```python
from build123d import *

# Parameters (mm, degrees)
BOSS_EXTRUDE1_DEPTH      = 5
BOSS_EXTRUDE1_DEPTH_BACK = 52.601
BOSS_EXTRUDE2_DEPTH      = 5
SKETCH3_W                = 4
SKETCH3_H                = 6
F_8_CLEARANCE_HOLE1_D    = 4.4958
CHAMFER1_SIZE            = 4
CUT_EXTRUDE7_DEPTH       = 189.558951211
BOSS_EXTRUDE10_START     = -5
BOSS_EXTRUDE10_DEPTH     = 5
CHAMFER4_SIZE            = 1


with BuildPart() as part:
    # Sketch1 → Boss-Extrude1 (new, two sides: drawn at the far end of the back side and taken through both)
    with BuildSketch(Plane(origin=(0, 0, 0), x_dir=(1, 0, 0), z_dir=(0, 1, 0)).offset(-BOSS_EXTRUDE1_DEPTH_BACK)):
        with BuildLine():
            Line((122.335390947, 32.191646773), (117.5, 30.919249667))
            ThreePointArc((117.5, 30.919249667), (83.736031712, 88.037077377), (25, 118.900168208))
            Line((25, 118.900168208), (26.028806584, 123.793179246))
            ThreePointArc((26.028806584, 123.793179246), (87.181958943, 91.660002372), (122.335390947, 32.191646773))
        make_face()
    extrude(amount=BOSS_EXTRUDE1_DEPTH + BOSS_EXTRUDE1_DEPTH_BACK)

    # Sketch2 → Boss-Extrude2 (add)
    with BuildSketch(Plane(origin=(0, 0, 0), x_dir=(1, 0, 0), z_dir=(0, 1, 0))):
        with BuildLine():
            Line((25, 118.900168208), (25, 84.894235624))
            ThreePointArc((25, 84.894235624), (25.761204675, 81.0674013), (27.928932188, 77.823167812))
            Line((27.928932188, 77.823167812), (43.071067812, 62.681032188))
            ThreePointArc((43.071067812, 62.681032188), (46.3153013, 60.513304675), (50.142135624, 59.7521))
            Line((50.142135624, 59.7521), (61, 59.7521))
            ThreePointArc((61, 59.7521), (63.773651249, 60.303813536), (66.125039239, 61.874960761))
            Line((66.125039239, 61.874960761), (81.125039239, 76.874960761))
            ThreePointArc((81.125039239, 76.874960761), (83.24659479, 82.137544003), (80.926866317, 87.315829447))
            ThreePointArc((80.926866317, 87.315829447), (60.589058557, 102.480133426), (37.5, 112.990980896))
            Line((37.5, 112.990980896), (37.5, 115.568161706))
            ThreePointArc((37.5, 115.568161706), (31.294377559, 117.400647073), (25, 118.900168208))
        make_face()
    extrude(amount=BOSS_EXTRUDE2_DEPTH)

    # Sweep1: sweep along a path in Sketch5
    with BuildLine(Plane.XZ.offset(52.601)) as sweep1_path:
        ThreePointArc((26.028806584, -123.793179246), (87.181958943, -91.660002372), (122.335390947, -32.191646773))
    # Sketch3 → Sweep1 (sweep)
    with BuildSketch(Plane(origin=(0, 0, 0), x_dir=(-0.20576131687242788, 0, 0.9786022074770342), z_dir=(-0.9786022074770342, 0, -0.20576131687242788))):
        with Locations((-128.5, -49.601)):
            Rectangle(SKETCH3_W, SKETCH3_H)
    sweep(path=sweep1_path.line)

    # #8 Clearance Hole1 (through all)
    with Locations(Plane(origin=(0, 5, 0), x_dir=(1, 0, 0), z_dir=(0, 1, 0))):
        with Locations((61, 67), (46, 52), (76, 52), (46, 82), (76, 82)):
            Hole(F_8_CLEARANCE_HOLE1_D / 2)

    # Chamfer1
    chamfer1_edges = [part.edges().sort_by_distance(p)[0] for p in [
        (87.181958943, -46.601, -91.660002372),
    ]]
    chamfer(chamfer1_edges, length=CHAMFER1_SIZE - 0.0001)  # a hair under: the kernel refuses the full size

    # Sketch21 → Cut-Extrude7 (cut, through all)
    with BuildSketch(Plane(origin=(0, 5, 0), x_dir=(1, 0, 0), z_dir=(0, 1, 0))):
        with BuildLine():
            ThreePointArc((46.481194337, 85.428989569), (44.410494667, 83.589505333), (42.571010431, 81.518805663))
            ThreePointArc((42.571010431, 81.518805663), (42.945660431, 78.361948651), (46.102517444, 78.736598651))
            ThreePointArc((46.102517444, 78.736598651), (47.589505333, 80.410494667), (49.263401349, 81.897482556))
            ThreePointArc((49.263401349, 81.897482556), (49.638051349, 85.054339569), (46.481194337, 85.428989569))
        make_face()
        with BuildLine():
            ThreePointArc((79.262817338, 81.727283432), (77.589505333, 83.589505333), (75.727283432, 85.262817338))
            ThreePointArc((75.727283432, 85.262817338), (72.566372961, 84.924064019), (72.90512628, 81.763153547))
            ThreePointArc((72.90512628, 81.763153547), (74.410494667, 80.410494667), (75.763153547, 78.90512628))
            ThreePointArc((75.763153547, 78.90512628), (78.924064019, 78.566372961), (79.262817338, 81.727283432))
        make_face()
    extrude(amount=-CUT_EXTRUDE7_DEPTH, mode=Mode.SUBTRACT)

    # Sketch32 → Boss-Extrude10 (add)
    with BuildSketch(Plane(origin=(0, 5, 0), x_dir=(1, 0, 0), z_dir=(0, 1, 0)).offset(BOSS_EXTRUDE10_START)):
        with BuildLine():
            Line((117.5, 30.919249667), (114.666962611, 30.173756984))
            ThreePointArc((114.666962611, 30.173756984), (105.505280532, 35.518247745), (110.849771294, 44.679929823))
            Line((110.849771294, 44.679929823), (112.783927672, 45.188888665))
            ThreePointArc((112.783927672, 45.188888665), (115.362808068, 38.127057514), (117.5, 30.919249667))
        make_face()
    extrude(amount=BOSS_EXTRUDE10_DEPTH)

    # Chamfer4
    chamfer4_edges = [part.edges().sort_by_distance(p)[0] for p in [
        (87.181958943, 5, -91.660002372),
        (44.410494667, 5, -83.589505333),
        (47.589505333, 5, -80.410494667),
        (49.638051349, 5, -85.054339569),
        (42.945660431, 5, -78.361948651),
        (74.410494667, 5, -80.410494667),
        (77.589505333, 5, -83.589505333),
        (121.851851852, -52.601, -32.064407063),
        (72.566372961, 5, -84.924064019),
        (78.924064019, 5, -78.566372961),
        (25.925925926, -52.601, -123.303878142),
        (83.736031712, -52.601, -88.037077377),
        (25.514403292, 5, -121.346673727),
        (111.816849483, 5, -44.934409244),
        (105.505280532, 5, -35.518247745),
        (82.973641884, 5, -88.755984319),
        (37.5, 5, -114.279571301),
        (25, 5, -101.897201916),
        (25.761204675, 5, -81.0674013),
        (35.5, 5, -70.2521),
        (46.3153013, 5, -60.513304675),
        (55.571067812, 5, -59.7521),
        (63.773651249, 5, -60.303813536),
        (73.625039239, 5, -69.374960761),
        (83.24659479, 5, -82.137544003),
        (60.589058557, 5, -102.480133426),
        (89.938700727, -52.601, -94.558342368),
        (118.501176779, 5, -31.182701878),
        (63.2479, 5, -67),
    ]]
    chamfer(chamfer4_edges, length=CHAMFER4_SIZE)


solid = part.part
```
Here's how the part is built. I have some questions about the finished solid (model axes, mm). A direction names the side the tool comes from. Give positions to 0.01 mm unless a question says otherwise; leave off trailing zeros. Loops run counter-clockwise (first coordinate to the right, second up) from the corner with the lowest first, then second, coordinate; pieces in that order, holes last. Notation, with made-up numbers: (-19.5, 24) -> (1.5, 24) arc R7 ccw to (1.5, 36) -> close; hole circle Ø8 at (47, -21.75). An arc over 180 degrees is marked (long way). Use one line per item in the form item = value. Start each with the question number.
1) Thinking about a two-plate mould opening in Z: for faces 1 (the face through (83.248, 1.972, -82.056)), 2 (the face through (25, 2, -102)), 3 (the face through (46.265, 1.972, -60.534)), which applies, +Z half, -Z half, draft (parallel to the pull), parting line (faces both ways), or undercut?
2) For P1, Ø2, axis at y = 3, z = -113.5, coming from the +X side; P2, Ø1.5, axis at y = -9.5, z = -82.5, coming from the +X side; P3, Ø6, axis at x = 61, z = -67, coming from the -Y side, each with a flat end and sliding along its axis, tell me the tip position at first contact or that it passes through.
3) Imagine slicing it at A-A (z = -67). Count the separate pieces of the cut face and the enclosed holes in it, then the cut area to 3 significant figures.
4) Imagine slicing it at B-B (y = -30). Please give me the cut outline in (x, z).
5) Which directions (+Z, -Z, +X, -X, +Y, -Y) give clear straight access to the entire face, cutting with the end or side of a thin tool? Please do faces 4 (the face through (47, 0, -90)), 5 (the face through (47.57, 2.03, -80.39)), 6 (the face through (63.509, 4.604, -60.848)).
6) Please list where these lines run through material, in increasing order: line 1 along Z through (x, y) = (61, 2.75); line 2 along X through (y, z) = (1.05, -67); line 3 along Y through (x, z) = (53.5, -101).
Check values:
q1.face_1 = undercut
q1.face_2 = draft
q1.face_3 = +Z half
q2.P1 = 57.84
q2.P2 = 96.54
q2.P3 = 0
q3.separate_pieces = 3
q3.enclosed_holes = 0
q3.area = 515 mm^2
q4.outline = (25, -118.9) -> (26.03, -123.79) arc R126.5 ccw to (122.34, -32.19) -> (117.5, -30.92) arc R121.5 cw to start
q5.face_4 = +Z, -X, -Y
q5.face_5 = +Y, -Y
q5.face_6 = +Z, +Y
q6.line_1 = -110.82 to -105.08, -102.24 to -69.25, -64.75 to -59.75
q6.line_2 = 38.75 to 58.75, 63.25 to 71.25, 101.36 to 107.3
q6.line_3 = 0 to 5
